Design review of the part shown in the three views and the two pictorial views. Dimensions are in mm from the part's minimum x, y and z. Give positions to 0.01 mm unless a question says otherwise; leave off trailing zeros. Order: outer loops, then holes, each group sorted by start corner. A loop starts at its lowest first (then second) coordinate and runs counter-clockwise, first axis right, second up. Notation, with made-up numbers: M 47.25,37.25 L 79.25,37.25 A31 ccw 79.25,70.25 Z; hole C 24.5,18.5 d2. An arc over 180 degrees is marked long. Answer as a JSON object with one key per item and string values.
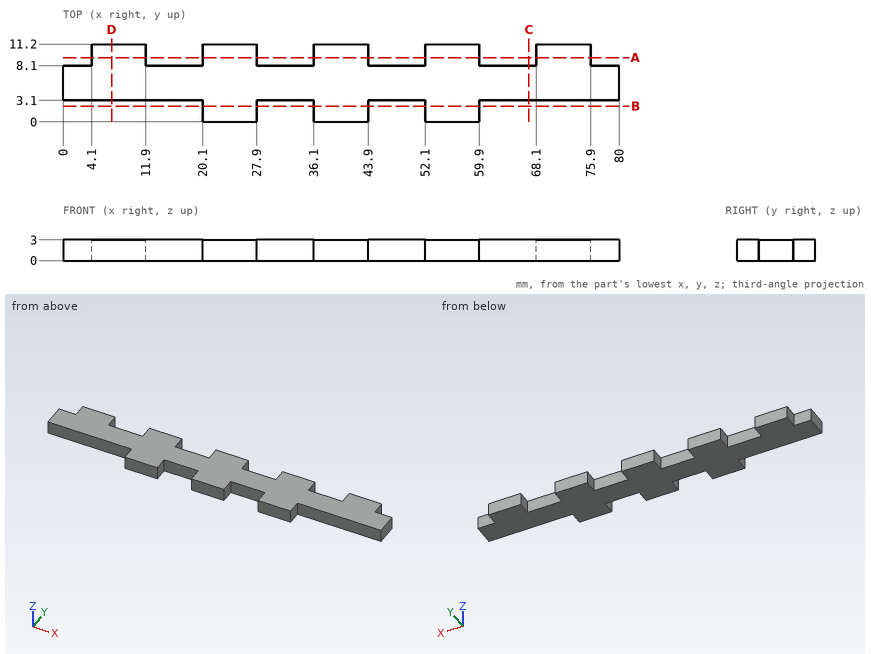
(1) To check wall thickness, follow L1, parallel to X at y = 9.75, z = 0.75; L2, parallel to X at y = 2.5, z = 1.9; L3, parallel to Y at x = 62, z = 2.05. State the ranges of each line that lie inside material, in increasing order. Write a range as from..to.
Checked values:
{"L1": "x = 4.1..11.9, 20.1..27.9, 36.1..43.9, 52.1..59.9, 68.1..75.9", "L2": "x = 20.1..27.9, 36.1..43.9, 52.1..59.9", "L3": "y = 3.1..8.1"}
(2) We need section D-D (x = 7). Write out the cut boundary in (y, z).
Checked values:
{"outline": "M 3.1,0 L 11.2,0 L 11.2,3 L 3.1,3 Z"}
(3) We need section B-B (y = 2.25). Write out the cut boundary in (x, z).
Checked values:
{"outline": "M 20.1,0 L 27.9,0 L 27.9,3 L 20.1,3 Z; M 36.1,0 L 43.9,0 L 43.9,3 L 36.1,3 Z; M 52.1,0 L 59.9,0 L 59.9,3 L 52.1,3 Z"}
(4) Insertion check: pin 1 (0.9 mm diameter, centred on y = 9, z = 1, fed in from -X); pin 2 (1.5 mm diameter, centred on x = 33.5, z = 2, fed in from -Y); pin 3 (0.9 mm diameter, centred on x = 78, z = 1, fed in from +Y). Each pin has a flat end and moves straight along its axis. Give the tip position at first contact, or say it passes through.
Checked values:
{"pin 1": "stops at x = 4.1", "pin 2": "stops at y = 3.1", "pin 3": "stops at y = 8.1"}
(5) We need section C-C (x = 67). Write out the cut boundary in (y, z).
Checked values:
{"outline": "M 3.1,0 L 8.1,0 L 8.1,3 L 3.1,3 Z"}
(6) We need section A-A (y = 9.25). Write out the cut boundary in (x, z).
Checked values:
{"outline": "M 4.1,0 L 11.9,0 L 11.9,3 L 4.1,3 Z; M 20.1,0 L 27.9,0 L 27.9,3 L 20.1,3 Z; M 36.1,0 L 43.9,0 L 43.9,3 L 36.1,3 Z; M 52.1,0 L 59.9,0 L 59.9,3 L 52.1,3 Z; M 68.1,0 L 75.9,0 L 75.9,3 L 68.1,3 Z"}
